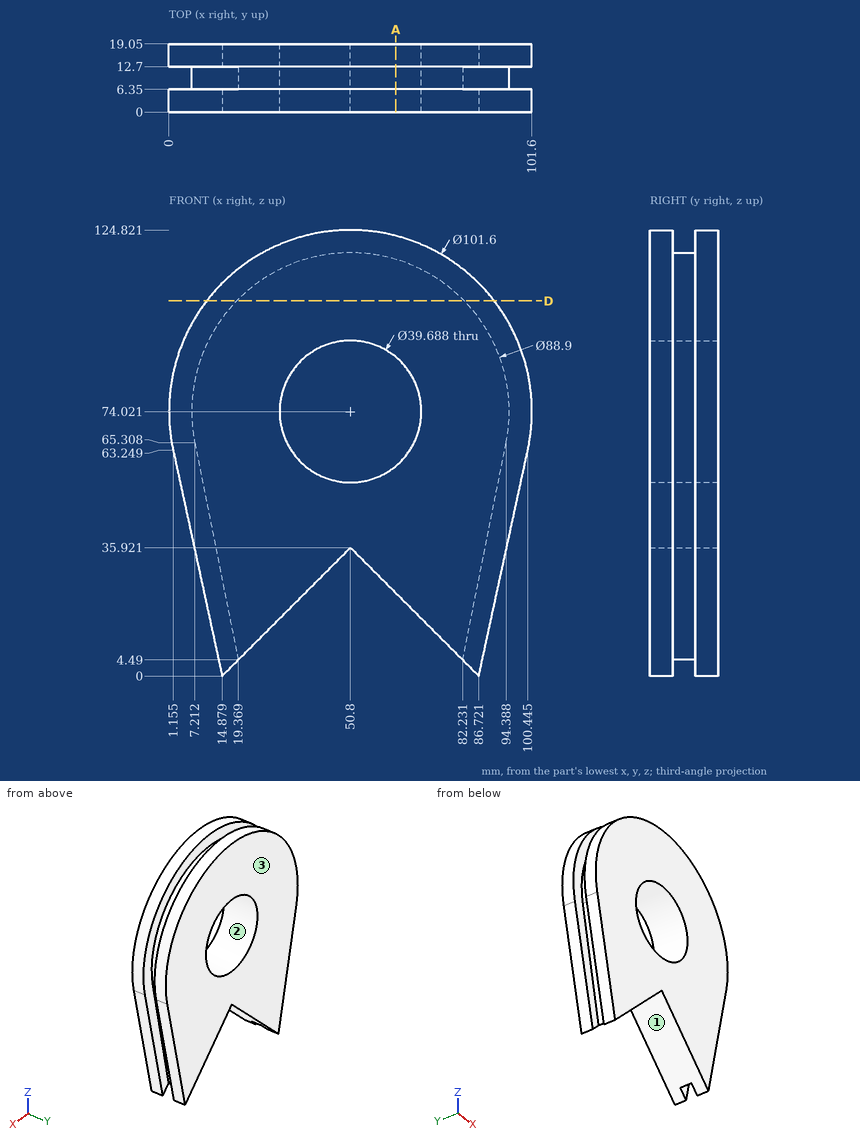
Verification items for this drawing (mm, ordinates from the low corner). Give positions to 0.01 mm unless a question says otherwise; leave off trailing zeros. Write each loop counter-clockwise with the first axis right and the second up, starting at its lowest first coordinate (ties: lowest second). Pieces come first, ordered by that corner, then holes. Notation, with made-up numbers: (51, 68.25) - (96, 68.25) arc R4 ccw to (96, 73.25) - close; hole circle Ø7 at (-15, 31.5). An arc over 180 degrees is marked (long way). Answer as CSV lines item,"result". Start each with the question number.
1. Draft check along Z on the marked faces 1, 2 and 3. Enter one of: pulls with the +Z half, pulls with the -Z half, needs draft (parallel to the pull), parting line crosses it, or undercut.
2. Thickness scan on line 1 (Z direction, x = 50.8, y = 4.25) (1 decimal); line 2 (Y direction, x = 9, z = 29.5); line 3 (Z direction, x = 50.8, y = 11.5) (1 decimal). Record the ranges inside material, lowest first.
3. Depth check by flat-ended pin: pin 1 (4 mm diameter, centred on y = 4, z = 67, fed in from +X); pin 2 (2 mm diameter, centred on x = 32.5, y = 16.5, fed in from -Z); pin 3 (1 mm diameter, centred on x = 56.5, y = 7.5, fed in from +Z). Enter the tip coordinate at first touch or a pass-through.
4. Sectioned sample at A-A (x = 63.5). Record the boundary of the cut face in (y, z).
5. Sectioned sample at D-D (z = 105). Record the boundary of the cut face in (x, y).
Derived:
1,face 1,"pulls with the -Z half"
1,face 2,"undercut"
1,face 3,"needs draft"
2,line 1,"35.9 to 54.2, 93.9 to 124.8"
2,line 2,"0 to 6.35, 12.7 to 19.05"
2,line 3,"35.9 to 54.2, 93.9 to 118.5"
3,pin 1,"x = 101.35"
3,pin 2,"z = 16.62"
3,pin 3,"z = 118.17"
4,outline,"(0, 23.22) - (19.05, 23.22) - (19.05, 58.77) - (0, 58.77) - close; (0, 89.27) - (19.05, 89.27) - (19.05, 123.21) - (12.7, 123.21) - (12.7, 116.62) - (6.35, 116.62) - (6.35, 123.21) - (0, 123.21) - close"
5,outline,"(10.54, 0) - (91.06, 0) - (91.06, 6.35) - (82.68, 6.35) - (82.68, 12.7) - (91.06, 12.7) - (91.06, 19.05) - (10.54, 19.05) - (10.54, 12.7) - (18.92, 12.7) - (18.92, 6.35) - (10.54, 6.35) - close"
